Check sheet for the drawn part. Datum: minimum x, y, z corner. Units: mm. Coordinates: 2 decimals unless noted, no trailing zeros. Write each loop counter-clockwise with the first axis right and the second up, starting at its lowest first coordinate (ties: lowest second). Pieces come first, ordered by that corner, then holes. Notation, with made-up numbers: M 29.25,18.5 L 43.25,18.5 A18 cw 43.25,46.5 Z; hole C -39,88.25 d3. An arc over 180 degrees is marked long. Answer in a Markdown table with one row per item.
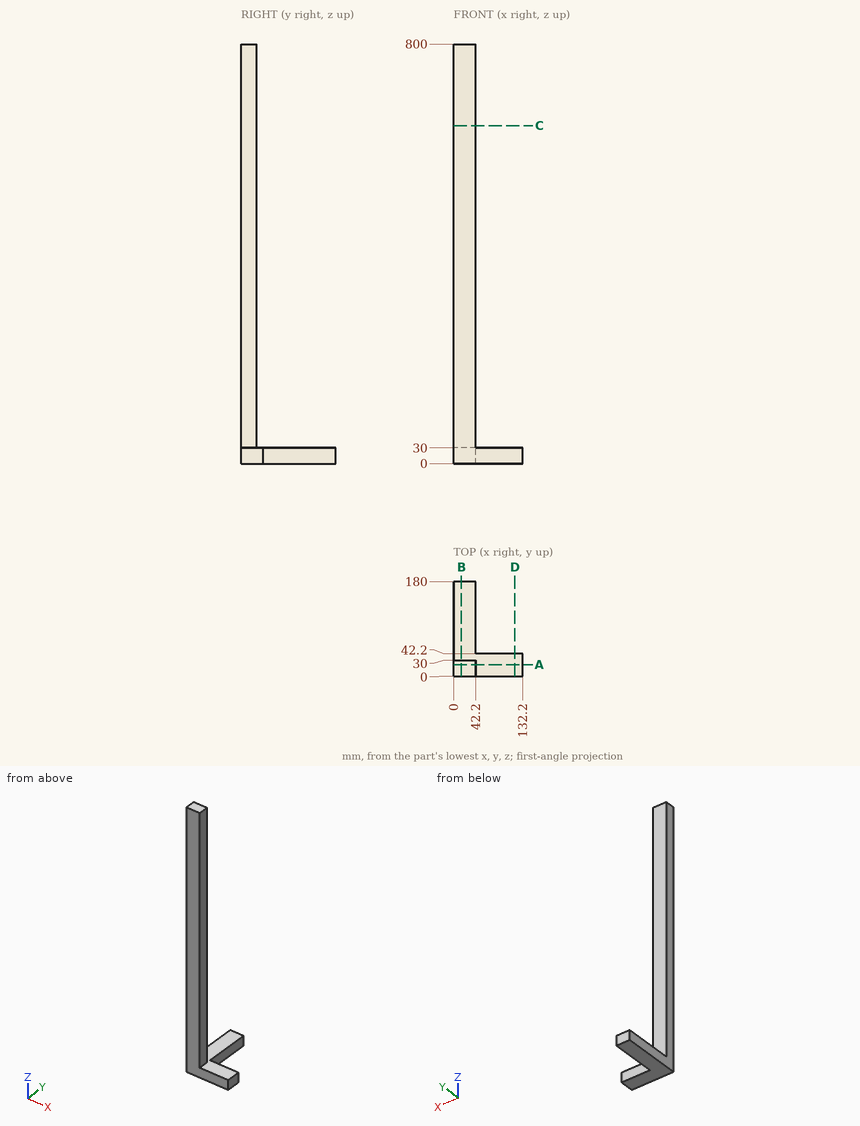
1) Sectioned sample at C-C (z = 644.5). Record the cut outline in (x, y).
Response values:
| item | result |
|---|---|
| outline | M 0,0 L 42.2,0 L 42.2,30 L 0,30 Z |
2) Thickness scan on L1, parallel to Y at x = 36, z = 486; L2, parallel to X at y = 15, z = 738. Record the ranges inside material, lowest first. Write a range as [from, to].
Response values:
| item | result |
|---|---|
| L1 | y = [0, 30] |
| L2 | x = [0, 42.2] |
3) Depth check by flat-ended pin: pin 1 (12 mm diameter, centred on x = 40.5, z = 256.5, fed in from +Y); pin 2 (15 mm diameter, centred on x = 105, z = 9, fed in from +Y); pin 3 (5 mm diameter, centred on x = 20.5, y = 90, fed in from +Z). Enter the tip coordinate at first touch or a pass-through.
Response values:
| item | result |
|---|---|
| pin 1 | stops at y = 30 |
| pin 2 | stops at y = 42.2 |
| pin 3 | stops at z = 30 |
4) Sectioned sample at A-A (y = 21.5). Record the cut outline in (x, z).
Response values:
| item | result |
|---|---|
| outline | M 0,0 L 132.2,0 L 132.2,30 L 42.2,30 L 42.2,800 L 0,800 Z |
5) Sectioned sample at B-B (x = 15). Record the cut outline in (y, z), then the cut area to 3 significant figures.
Response values:
| item | result |
|---|---|
| outline | M 0,0 L 180,0 L 180,30 L 30,30 L 30,800 L 0,800 Z |
| area | 28,500 mm² |
